Geometry: final body of the model. Coordinates: model frame, mm. Coordinates: 2 decimals unless noted, no trailing zeros. Loops run counter-clockwise (first coordinate to the right, second up) from the corner with the lowest first, then second, coordinate; pieces in that order, holes last. Notation, with made-up numbers: (79, 21.5) - (104, 21.5) arc R5 cw to (104, 25.5) - close; hole circle Ø10 at (3.5, 70). An arc over 180 degrees is marked (long way). Answer in a Markdown table with one row per item.
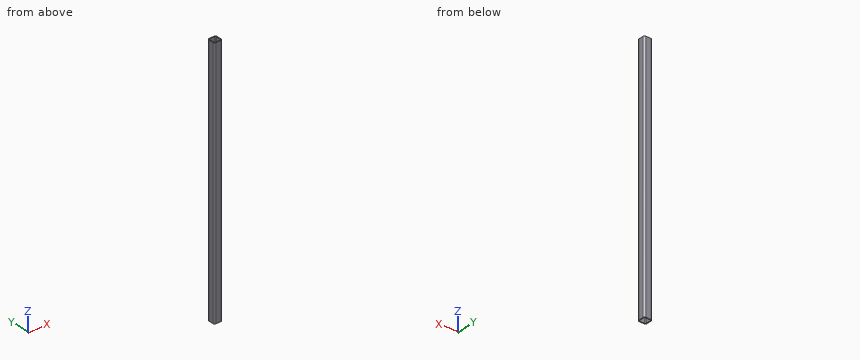
Autodesk Inventor part; units mm, degrees
ref_plane "Start Plane" through (0, 0, 15) normal (0, 0, 1) x (1, 0, 0)
ref_plane "End Plane" through (0, 0, 935) normal (0, 0, 1) x (1, 0, 0)
ref_plane "Work Plane4" through (-1731, 0, 15) normal (0, 0, -1) x (-1, 0, 0)
ref_plane "Start Plane" through (0, 0, 15) normal (0, 0, 1) x (1, 0, 0)
ref_plane "End Plane" through (0, 0, 935) normal (0, 0, 1) x (1, 0, 0)
sketch "Sketch" plane through (0, 0, 0) normal (0, 0, 1) x (1, 0, 0)
  line L0 (-15, -9) -> (-15, 9)
  line L1 (-9, 15) -> (9, 15)
  line L2 (15, 9) -> (15, -9)
  line L3 (9, -15) -> (-9, -15)
  arc A0 (-15, -9) -> (-9, -15) centre (-9, -9) ccw
  arc A1 (-9, 15) -> (-15, 9) centre (-9, 9) ccw
  arc A2 (15, 9) -> (9, 15) centre (9, 9) ccw
  arc A3 (9, -15) -> (15, -9) centre (9, -9) ccw
  arc A4 (-9, 12) -> (-12, 9) centre (-9, 9) ccw
  line L4 (-9, 12) -> (9, 12)
  arc A5 (12, 9) -> (9, 12) centre (9, 9) ccw
  line L5 (12, 9) -> (12, -9)
  arc A6 (9, -12) -> (12, -9) centre (9, -9) ccw
  line L6 (9, -12) -> (-9, -12)
  arc A7 (-12, -9) -> (-9, -12) centre (-9, -9) ccw
  line L7 (-12, -9) -> (-12, 9)
  line L8 (0, 22.7397) -> (0, -22.7397) construction
  line L9 (-22.7397, 0) -> (22.7397, 0) construction
  dimension "d7" = 6
  dimension "d10" = 30
  dimension "d11" = 30
  dimension "d12" = 3
  dimension "d15" = 15
  dimension "d16" = 15
extrude "Body" add sketch "Sketch" along normal up to surface (920 mm away) from surface at 15
sketch "Sketch3" plane through (0, 0, 0) normal (0, 0, 1) x (1, 0, 0)
  line L0 (0, 0) -> (10, 0)
ref_plane "Work Plane3" through (0, 0, 0) normal (0, -1, 0) x (1, 0, 0)
ref_plane "Work Plane4" through (-1731, 0, 15) normal (0, 0, -1) x (-1, 0, 0)
split "Split1" plane through (-1731, 0, 15) removes the side toward (0, 0, -1)
ref_plane "Work Plane5" through (0, -991, 935) normal (0, 0, 1) x (1, 0, 0)
split "Split2" plane through (0, -991, 935) removes the side toward (0, 0, 1)
sketch "Sketch4" plane through (0, 0, 0) normal (0, -1, 0) x (1, 0, 0)
  line L0 (-2, 15) -> (12, 15)
  line L1 (-2, 935) -> (12, 935)
  dimension "d18" = 920
equation "\"d7\" = G_IR"
equation "\"d10\" = G_H"
equation "\"d11\" = G_W"
equation "\"d12\" = G_T"
equation "\"d15\" = 0.5 * d10"
equation "\"d16\" = 0.5 * d11"
equation "\"d3\" = G_L"
equation "\"G_W\" = 30"
equation "\"G_H\" = 30"
equation "\"G_T\" = 3"
equation "\"G_IR\" = 6"
equation "\"G_L\" = d18"
equation "\"G_OFFSET_START\" = -15"
equation "\"G_OFFSET_END\" = -15"
equation "\"d13\" = -G_OFFSET_START"
equation "\"d14\" = G_OFFSET_END + B_L"
properties part number "DIN EN 10219-2 - 30 x 30 x 3  - 920" material "Steel, Mild"
(1) Cut plane A-A on z = 289.5. Output: boundary loops of the cut face in (x, y), then the cut area to 3 significant figures.
Verdict:
| item | result |
|---|---|
| outline | (-15, -9) arc R6 ccw to (-9, -15) - (9, -15) arc R6 ccw to (15, -9) - (15, 9) arc R6 ccw to (9, 15) - (-9, 15) arc R6 ccw to (-15, 9) - close; hole (-12, -9) arc R3 ccw to (-9, -12) - (9, -12) arc R3 ccw to (12, -9) - (12, 9) arc R3 ccw to (9, 12) - (-9, 12) arc R3 ccw to (-12, 9) - close |
| area | 301 mm² |
(2) First-contact query: pin 1 Ø1 at (x, y) = (10, 6) entering from -Z; pin 2 Ø2 at (y, z) = (-11.5, 707) entering from -X. Flat tips, straight axial feed; report the tip coordinate or a pass-through.
Verdict:
| item | result |
|---|---|
| pin 1 | passes through |
| pin 2 | stops at x = -14.81 |
(3) Cut plane B-B on x = -0.25. Output: boundary loops of the cut face in (y, z).
Verdict:
| item | result |
|---|---|
| outline | (-15, 15) - (-12, 15) - (-12, 935) - (-15, 935) - close; (12, 15) - (15, 15) - (15, 935) - (12, 935) - close |
(4) Ray query, probe 1 along X at (y, z) = (8.25, 52); probe 2 along Y at (x, z) = (9.25, 171); probe 3 along Y at (x, z) = (-10, 401). Return the intervals inside material, ascending.
Verdict:
| item | result |
|---|---|
| probe 1 | x = -15 to -12, 12 to 15 |
| probe 2 | y = -14.99 to -11.99, 11.99 to 14.99 |
| probe 3 | y = -14.92 to -11.83, 11.83 to 14.92 |
